Could you check a few things on this model? Use its own coordinates, in mm. Give positions to 0.01 mm unless a question says otherwise; leave off trailing zeros. Loops run counter-clockwise (first coordinate to the right, second up) from the corner with the lowest first, then second, coordinate; pieces in that order, holes last. Notation, with made-up numbers: M 24.25,63.25 L 49.25,63.25 A11 cw 49.25,83.25 Z; hole C 63.5,78.5 d10. An arc over 180 degrees is marked long. Return JSON: item names as keys, results as strings. Group by question number.
1. If we section it at D-D (y = -11): Write out the boundary of the cut face in (x, z).
2. Please list where these lines run through material, in increasing order: line 1 (Y direction, x = 20, z = 0.35); line 2 (X direction, y = -18, z = 2.3); line 3 (X direction, y = -11, z = 0.35).
3. If we section it at C-C (x = -2.5): Write out the boundary of the cut face in (y, z), plus the area to 3 significant figures.
4. If we mould it in two halves opening along X, with no side actions, what happens to faces 1 (the cylindrical face through (-9.94, 10.37, 1.48)), 2 (the flat face through (-25, 0, 1)), 3 (the flat face through (24.2, 0.3, 2.3)), 4 (the conical face through (20, -22, 2))? For each: +X half, -X half, draft (parallel to the pull), parting line (faces both ways), or undercut.
5. If we section it at A-A (y = 0): Write out the boundary of the cut face in (x, z), plus the area to 4 significant figures.
6. For pin 1 (2.5 mm diameter, centred on x = 20, y = 20, fed in from -Z); pin 2 (4 mm diameter, centred on x = -20, y = 20, fed in from +Z), each with a flat end and sliding along its axis, tell me the tip position at first contact or that it passes through.
7. If we section it at B-B (z = 2.3): Write out the boundary of the cut face in (x, y), plus the area to 3 significant figures.
```python
from build123d import *

# Parameters (mm, degrees)
SKETCH_R     = 1.5
SKETCH_R_2   = 12.5
PAD_DEPTH    = 3
CHAMFER_SIZE = 1.5


with BuildPart() as part:
    # Sketch → Pad (new body)
    with BuildSketch(Plane.XY):
        with BuildLine():
            Line((-20, 25), (20, 25))
            ThreePointArc((25, 20), (23.535534, 23.535534), (20, 25))
            Line((25, 20), (25, -20))
            ThreePointArc((20, -25), (23.535534, -23.535534), (25, -20))
            Line((20, -25), (-20, -25))
            ThreePointArc((-25, -20), (-23.535534, -23.535534), (-20, -25))
            Line((-25, -20), (-25, 20))
            ThreePointArc((-20, 25), (-23.535534, 23.535534), (-25, 20))
        make_face()
        with Locations((-9.616538, 11.835739)):
            Circle(SKETCH_R, mode=Mode.SUBTRACT)
        with Locations((9.616538, -11.835739)):
            Circle(SKETCH_R, mode=Mode.SUBTRACT)
        with Locations((-20, 20)):
            Circle(SKETCH_R, mode=Mode.SUBTRACT)
        with Locations((20, 20)):
            Circle(SKETCH_R, mode=Mode.SUBTRACT)
        with Locations((20, -20)):
            Circle(SKETCH_R, mode=Mode.SUBTRACT)
        with Locations((-20, -20)):
            Circle(SKETCH_R, mode=Mode.SUBTRACT)
        Circle(SKETCH_R_2, mode=Mode.SUBTRACT)
    extrude(amount=PAD_DEPTH)

    # Chamfer
    chamfer_edges = [part.edges().sort_by_distance(p)[0] for p in [
        (0, 25, 3),
        (-21.5, 20, 3),
        (18.5, 20, 3),
        (18.5, -20, 3),
        (-21.5, -20, 3),
    ]]
    chamfer(chamfer_edges, length=CHAMFER_SIZE)


solid = part.part
```
Answer:
{
 "1": {"outline": "M -25,0 L -5.94,0 L -5.94,3 L -23.5,3 L -25,1.5 Z; M 5.94,0 L 8.37,0 L 8.37,3 L 5.94,3 Z; M 10.86,0 L 25,0 L 25,1.5 L 23.5,3 L 10.86,3 Z"},
 "2": {"line 1": "y = -25 to -21.5, -18.5 to 18.5, 21.5 to 25", "line 2": "x = -24.2 to -21.14, -18.86 to 18.86, 21.14 to 24.2", "line 3": "x = -25 to -5.94, 5.94 to 8.37, 10.86 to 25"},
 "3": {"outline": "M -25,0 L -12.25,0 L -12.25,3 L -23.5,3 L -25,1.5 Z; M 12.25,0 L 25,0 L 25,1.5 L 23.5,3 L 12.25,3 Z", "area": "74.3 mm²"},
 "4": {"face 1": "undercut", "face 2": "-X half", "face 3": "+X half", "face 4": "undercut"},
 "5": {"outline": "M -25,0 L -12.5,0 L -12.5,3 L -23.5,3 L -25,1.5 Z; M 12.5,0 L 25,0 L 25,1.5 L 23.5,3 L 12.5,3 Z", "area": "72.75 mm²"},
 "6": {"pin 1": "passes through", "pin 2": "stops at z = 2"},
 "7": {"outline": "M -24.2,-20 A4.2 ccw -20,-24.2 L 20,-24.2 A4.2 ccw 24.2,-20 L 24.2,20 A4.2 ccw 20,24.2 L -20,24.2 A4.2 ccw -24.2,20 Z; hole C -20,-20 d4.6; hole C -20,20 d4.6; hole C 0,0 d25; hole C -9.62,11.84 d3; hole C 9.62,-11.84 d3; hole C 20,-20 d4.6; hole C 20,20 d4.6", "area": "1,760 mm²"}
}
